```python
from build123d import *

# Parameters (mm, degrees)
F0_W      = 76
F0_H      = 44
F1_DEPTH  = 36
F2_W      = 11
F2_H      = 37
F3_DEPTH  = 36
F4_W      = 7
F4_H      = 18
F4_W_2    = 40
F4_H_2    = 36
F5_DEPTH  = 29
F6_R      = 15
F7_DEPTH  = 22
F9_DEPTH  = 7
F11_DEPTH = 22


with BuildPart() as f1:
    # F0 (on Front) → F1 (new body)
    with BuildSketch(Plane.XZ):
        with Locations((38, 22)):
            Rectangle(F0_W, F0_H)
    extrude(amount=-F1_DEPTH)

    # F2 (on face) → F3 (cut)
    with BuildSketch(Plane.XZ):
        with Locations((5.5, 18.5)):
            Rectangle(F2_W, F2_H)
        with Locations((70.5, 18.5)):
            Rectangle(F2_W, F2_H)
    extrude(amount=-F3_DEPTH, mode=Mode.SUBTRACT)

    # F4 (on face) → F5 (cut)
    with BuildSketch(Plane.XY.offset(44)):
        with Locations((72.5, 18)):
            Rectangle(F4_W, F4_H)
        with Locations((38, 18)):
            Rectangle(F4_W_2, F4_H_2)
        with Locations((3.5, 18)):
            Rectangle(F4_W, F4_H)
    extrude(amount=-F5_DEPTH, mode=Mode.SUBTRACT)

    # F6 (on face) → F7 (join)
    with BuildSketch(Plane.XY.offset(15)):
        with Locations((38, 18)):
            Circle(F6_R)
    extrude(amount=F7_DEPTH)

    # F8 (on face) → F9 (cut)
    with BuildSketch(Plane.XY.offset(37)):
        with BuildLine():
            Line((43, 18), (38, 18))
            Line((38, 18), (38, 3))
            ThreePointArc((38, 3), (40.5365296809, 3.2160216052), (43, 3.8578643763))
            Line((43, 3.8578643763), (43, 18))
        make_face()
        with BuildLine():
            Line((38, 3), (38, 18))
            Line((38, 18), (43, 18))
            Line((43, 18), (43, 32.1421356237))
            ThreePointArc((43, 32.1421356237), (38, 33), (33, 32.1421356237))
            Line((33, 32.1421356237), (33, 3.8578643763))
            ThreePointArc((33, 3.8578643763), (35.4634703191, 3.2160216052), (38, 3))
        make_face()
        with BuildLine():
            ThreePointArc((33, 32.1421356237), (38, 33), (43, 32.1421356237))
            Line((43, 32.1421356237), (43, 36))
            Line((43, 36), (33, 36))
            Line((33, 36), (33, 32.1421356237))
        make_face()
        with BuildLine():
            ThreePointArc((43, 3.8578643763), (40.5365296809, 3.2160216052), (38, 3))
            Line((38, 3), (38, 0))
            Line((38, 0), (43, 0))
            Line((43, 0), (43, 3.8578643763))
        make_face()
        with BuildLine():
            Line((38, 0), (38, 3))
            ThreePointArc((38, 3), (35.4634703191, 3.2160216052), (33, 3.8578643763))
            Line((33, 3.8578643763), (33, 0))
            Line((33, 0), (38, 0))
        make_face()
    extrude(amount=-F9_DEPTH, mode=Mode.SUBTRACT)

    # F10 (on face) → F11 (cut)
    with BuildSketch(Plane.XY.offset(37)):
        with BuildLine():
            ThreePointArc((33, 9.3397459622), (43, 9.3397459622), (48, 18))
            ThreePointArc((48, 18), (43, 26.6602540378), (33, 26.6602540378))
            Line((33, 26.6602540378), (33, 9.3397459622))
        make_face()
        with BuildLine():
            Line((33, 9.3397459622), (33, 26.6602540378))
            ThreePointArc((33, 26.6602540378), (28, 18), (33, 9.3397459622))
        make_face()
    extrude(amount=-F11_DEPTH, mode=Mode.SUBTRACT)


solid = f1.part
```
Work out the finished part from the listing and answer in its coordinate system (mm). A direction names the side the tool comes from. Give positions to 0.01 mm unless a question says otherwise; leave off trailing zeros. Loops run counter-clockwise (first coordinate to the right, second up) from the corner with the lowest first, then second, coordinate; pieces in that order, holes last. Notation, with made-up numbers: M 58,22 L 80,22 A22 cw 80,40 Z; hole C 68,81 d10. An arc over 180 degrees is marked long. One line per item, written item: value. Start each with the question number.
1. Find section D-D (z = 5). Give the vertices of the cut face in (x, y).
2. Find section B-B (x = 38). Give the vertices of the cut face in (y, z), and give its area (3 significant figures).
3. Which of the six approach directions +Z, -Z, +X, -X, +Y, -Y give full straight-line access (tool end or side, diameter ignored) to faces 1 (the face through (3, 27, 41)), 2 (the face through (8, 18, 37)), 3 (the face through (43, 7, 34)), 4 (the face through (72, 9, 41)), 5 (the face through (28.8, 30.3, 15))?
4. Find section A-A (z = 25). Give the vertices of the cut face in (x, y).
5. Find section C-C (y = 25.5). Give the vertices of the cut face in (x, z).
6. Determine the mould class of faces 6 (the face through (51.856, 12.255, 25.846)), 7 (the face through (58, 18, 30)), 8 (the face through (7, 18, 41)) for opening direction Y: released by +Y, released by -Y, zero draft, split by the parting line, or undercut.
7. Find the intervals of material crossed by probe 1 along X at (y, z) = (2, 32.5); probe 2 along X at (y, z) = (15, 15.5); probe 3 along X at (y, z) = (5, 17), in increasing order.
8. Each of these flat-tipped pins is pushed along its axis until it touches: P1, Ø3, axis at y = 6, z = 7, coming from the -X side; P2, Ø3.5, axis at x = 70, y = 16, coming from the -Z side; P3, Ø2, axis at x = 3.5, z = 40, coming from the -Y side; P4, Ø12, axis at x = 42, z = 30, coming from the +Y side. Where does it stop, or does it pass through?
Reported:
1. outline: M 11,0 L 65,0 L 65,36 L 11,36 Z
2. outline: M 0,0 L 36,0 L 36,15 L 33,15 L 33,30 L 28,30 L 28,15 L 8,15 L 8,30 L 3,30 L 3,15 L 0,15 Z
2. area: 690 mm²
3. face 1: +Z, -Z, -X
3. face 2: -Z, -X, +Y, -Y
3. face 3: +Z, +Y, -Y
3. face 4: +Z, -Z, +X
3. face 5: +Z
4. outline: M 11,0 L 18,0 L 18,36 L 11,36 Z; C 38,18 d30; M 58,0 L 65,0 L 65,36 L 58,36 Z; hole C 38,18 d20
5. outline: M 7,37 L 11,37 L 11,0 L 65,0 L 65,37 L 69,37 L 69,44 L 58,44 L 58,15 L 50.99,15 L 50.99,37 L 44.61,37 L 44.61,15 L 31.39,15 L 31.39,37 L 25.01,37 L 25.01,15 L 18,15 L 18,44 L 7,44 Z
6. face 6: split by the parting line
6. face 7: zero draft
6. face 8: undercut
7. probe 1: x = 11 to 18, 58 to 65
7. probe 2: x = 11 to 18, 23.3 to 28.46, 47.54 to 52.7, 58 to 65
7. probe 3: x = 11 to 18, 30.52 to 45.48, 58 to 65
8. P1: stops at x = 11
8. P2: stops at z = 37
8. P3: stops at y = 0
8. P4: stops at y = 33
